```python
from build123d import *

# Parameters (mm, degrees)
ESQUISSE1_R        = 4
ESQUISSE1_R_2      = 0.875
ESQUISSE1_R_3      = 1.5
BOSS_EXTRU_1_DEPTH = 5


with BuildPart() as part:
    # Esquisse1 → Boss.-Extru.1 (new body)
    with BuildSketch(Plane.XY):
        with BuildLine():
            Line((-9.768700016, 3.85), (-4.651761912, 16.833333333))
            ThreePointArc((-4.651761912, 16.833333333), (0, 20), (4.651761912, 16.833333333))
            Line((4.651761912, 16.833333333), (9.768700016, 3.85))
            ThreePointArc((9.768700016, 3.85), (10.5, 0), (9.768700016, -3.85))
            Line((9.768700016, -3.85), (4.651761912, -16.833333333))
            ThreePointArc((4.651761912, -16.833333333), (0, -20), (-4.651761912, -16.833333333))
            Line((-4.651761912, -16.833333333), (-9.768700016, -3.85))
            ThreePointArc((-9.768700016, -3.85), (-10.5, 0), (-9.768700016, 3.85))
        make_face()
        Circle(ESQUISSE1_R, mode=Mode.SUBTRACT)
        with Locations((7.25, 3.65)):
            Circle(ESQUISSE1_R_2, mode=Mode.SUBTRACT)
        with Locations((3.65, -7.25)):
            Circle(ESQUISSE1_R_2, mode=Mode.SUBTRACT)
        with Locations((-7.25, -3.65)):
            Circle(ESQUISSE1_R_2, mode=Mode.SUBTRACT)
        with Locations((-3.65, 7.25)):
            Circle(ESQUISSE1_R_2, mode=Mode.SUBTRACT)
        with Locations((0, 15)):
            Circle(ESQUISSE1_R_3, mode=Mode.SUBTRACT)
        with Locations(Location((0, -15, 0), (0, 0, 180))):
            Circle(ESQUISSE1_R_3, mode=Mode.SUBTRACT)
    extrude(amount=BOSS_EXTRU_1_DEPTH)


solid = part.part
```
Geometry check sheet. Reference: the model listing, model coordinates, mm. Coordinates: 2 decimals unless noted, no trailing zeros. Loops run counter-clockwise (first coordinate to the right, second up) from the corner with the lowest first, then second, coordinate; pieces in that order, holes last. Notation, with made-up numbers: (54, -3) -> (107, -3) arc R31 ccw to (107, 22) -> close; hole circle Ø10 at (-23.75, -29.5). An arc over 180 degrees is marked (long way). Put each result on its own line as item: value.
1) Cross-section at D-D on x = -7. Record the boundary of the cut face in (y, z), plus the area to 3 significant figures.
Result set:
outline: (-10.88, 0) -> (-4.49, 0) -> (-4.49, 5) -> (-10.88, 5) -> close; (-2.81, 0) -> (10.88, 0) -> (10.88, 5) -> (-2.81, 5) -> close
area: 100 mm^2
2) Cross-section at B-B on y = 0. Record the boundary of the cut face in (x, z), plus the area to 3 significant figures.
Result set:
outline: (-10.5, 0) -> (-4, 0) -> (-4, 5) -> (-10.5, 5) -> close; (4, 0) -> (10.5, 0) -> (10.5, 5) -> (4, 5) -> close
area: 65.0 mm^2
3) Cross-section at C-C on z = 2.2. Record the boundary of the cut face in (x, y) (3 decimals).
Result set:
outline: (-9.769, -3.85) -> (-4.652, -16.833) arc R5 ccw to (4.652, -16.833) -> (9.769, -3.85) arc R10.5 ccw to (9.769, 3.85) -> (4.652, 16.833) arc R5 ccw to (-4.652, 16.833) -> (-9.769, 3.85) arc R10.5 ccw to start; hole circle Ø1.75 at (-7.25, -3.65); hole circle Ø1.75 at (-3.65, 7.25); hole circle Ø8 at (0, 0); hole circle Ø3 at (0, -15); hole circle Ø3 at (0, 15); hole circle Ø1.75 at (3.65, -7.25); hole circle Ø1.75 at (7.25, 3.65)
4) Gauge pin test, flat ends, axial feed: pin 1 Ø2 at (x, z) = (2.5, 2.5) entering from +Y; pin 2 Ø1.5 at (y, z) = (6.5, 0.5) entering from +X; pin 3 Ø1.1 at (x, y) = (3.65, -7.25) entering from +Z; pin 4 Ø1.5 at (x, z) = (-4, 1.5) entering from -Y. Record the tip position at first contact, or that the pin passes through.
Result set:
pin 1: stops at y = 19.77
pin 2: stops at x = 9.02
pin 3: passes through
pin 4: stops at y = -18.8
5) Thickness scan on line 1 (Y direction, x = 3.65, z = 1.25) (3 decimals); line 2 (X direction, y = 16, z = 3.9); line 3 (X direction, y = -3.5, z = 0.3). Record the ranges inside material, lowest first.
Result set:
line 1: y = -18.417 to -8.125, -6.375 to -1.636, 1.636 to 18.417
line 2: x = -4.98 to -1.12, 1.12 to 4.98
line 3: x = -9.9 to -8.11, -6.39 to -1.94, 1.94 to 9.9
6) Release check for a two-part mould opening along Y. For faces 1 (the flat face through (-7.174, -10.433, 2.465)), 2 (the cylindrical face through (3.54, -6.38, 2.46)), 3 (the cylindrical face through (0, 20, 2)), 4 (the cylindrical face through (-0.867, -3.905, 2.465)) record: released by +Y, released by -Y, zero draft, split by the parting line, or undercut.
Result set:
face 1: released by -Y
face 2: undercut
face 3: released by +Y
face 4: undercut
7) Cross-section at A-A on x = 0. Record the boundary of the cut face in (y, z).
Result set:
outline: (-20, 0) -> (-16.5, 0) -> (-16.5, 5) -> (-20, 5) -> close; (-13.5, 0) -> (-4, 0) -> (-4, 5) -> (-13.5, 5) -> close; (4, 0) -> (13.5, 0) -> (13.5, 5) -> (4, 5) -> close; (16.5, 0) -> (20, 0) -> (20, 5) -> (16.5, 5) -> close
